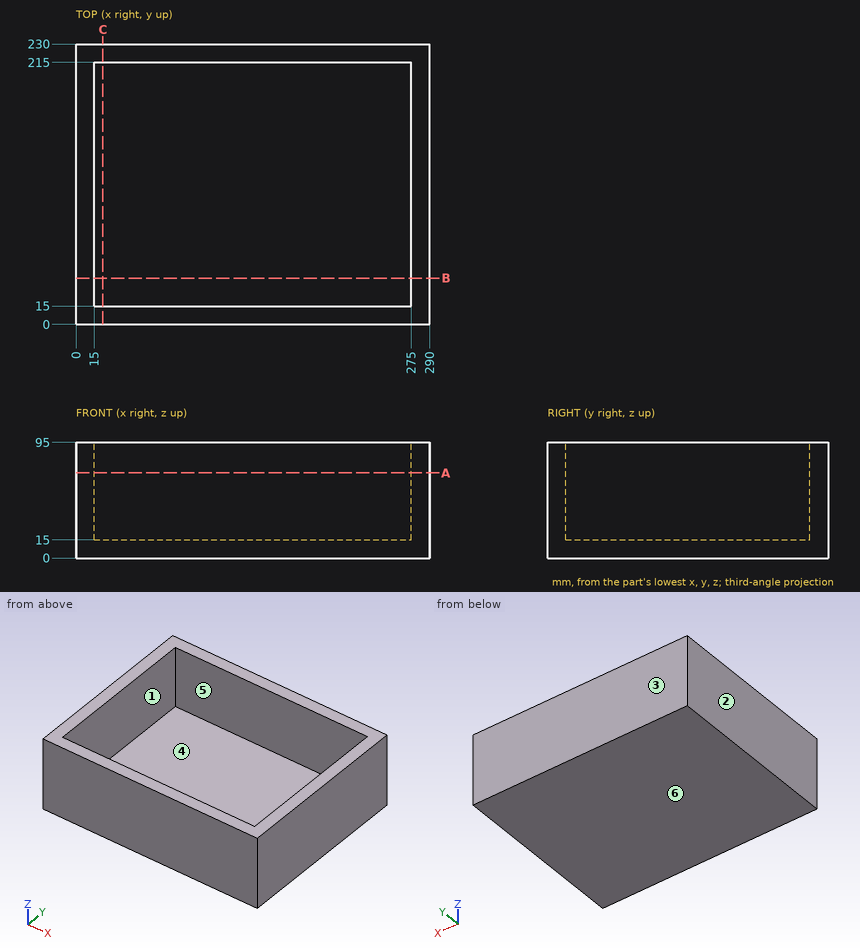
Could you check a few things on this drawing? It's one solid part, dimensions in mm from its lowest x, y, z. A direction names the side the tool comes from. Coordinates: 2 decimals unless noted, no trailing zeros. Write each loop counter-clockwise with the first axis right and the second up, starting at its lowest first coordinate (ties: lowest second). Pieces come first, ordered by that corner, then holes.
Q1. Imagine slicing it at C-C, the plane x = 22. List the corners of the cut face in (y, z) for me, plus the area to 3 significant figures.
Results found:
outline: (0, 0) - (230, 0) - (230, 95) - (215, 95) - (215, 15) - (15, 15) - (15, 95) - (0, 95) - close
area: 5,850 mm2
Q2. Imagine slicing it at A-A, the plane z = 70. List the corners of the cut face in (x, y) for me.
Results found:
outline: (0, 0) - (290, 0) - (290, 230) - (0, 230) - close; hole (15, 15) - (275, 15) - (275, 215) - (15, 215) - close
Q3. Which directions (+Z, -Z, +X, -X, +Y, -Y) give clear straight access to the entire face, cutting with the end or side of a thin tool? Please do the marked faces 1 and 2.
Results found:
face 1: +Z
face 2: +Z, -Z, -X, +Y, -Y
Q4. Imagine slicing it at B-B, the plane y = 38. List the corners of the cut face in (x, z) for me.
Results found:
outline: (0, 0) - (290, 0) - (290, 95) - (275, 95) - (275, 15) - (15, 15) - (15, 95) - (0, 95) - close
Q5. For P1, Ø1, axis at x = 73.5, z = 51.5, coming from the -Y side, with a flat end and sliding along its axis, tell me the tip position at first contact or that it passes through.
Results found:
P1: stops at y = 0
Q6. If we mould it in two halves opening along Y, with no side actions, what happens to the marked faces 3, 4, 5 and 6? For each: +Y half, -Y half, draft (parallel to the pull), parting line (faces both ways), or undercut.
Results found:
face 3: +Y half
face 4: undercut
face 5: undercut
face 6: draft
Q7. Please list where these lines run through material, in increasing order: L1, parallel to Y at x = 121.5, z = 28.5; L2, parallel to X at y = 183, z = 66; L3, parallel to Z at x = 132.5, y = 101.
Results found:
L1: y = 0 to 15, 215 to 230
L2: x = 0 to 15, 275 to 290
L3: z = 0 to 15
